Verification items for this drawing (mm, ordinates from the low corner). A direction names the side the tool comes from. Give positions to 0.01 mm unless a question says otherwise; leave off trailing zeros. Order: outer loops, then holes, each group sorted by start corner. A loop starts at its lowest first (then second) coordinate and runs counter-clockwise, first axis right, second up.
(1) Mould release check, pull along X, two halves, no side actions. Record for the marked faces 1, 2 and 3: pulls with the +X half, pulls with the -X half, needs draft (parallel to the pull), parting line crosses it, or undercut.
(2) Access from +Z, -Z, +X, -X, +Y, -Y to the whole of each face (thin tool, end or side, straight path). Record for the marked faces 4, 5 and 6.
(3) Gauge pin test, flat ends, axial feed: pin 1 (10 mm diameter, centred on x = 6.5, z = 13.5, fed in from -Y); pin 2 (1.2 mm diameter, centred on x = 13.5, y = 23.5, fed in from +Z); pin 3 (2 mm diameter, centred on x = 1, y = 33, fed in from +Z). Record the tip position at first contact, or that the pin passes through.
(4) Sectioned sample at B-B on z = 19. Record the cut outline in (x, y).
(5) Sectioned sample at A-A on y = 29. Record the cut outline in (x, z), plus the area to 3 significant figures.
(6) Sectioned sample at C-C on y = 24. Record the cut outline in (x, z).
(7) Scan lines: L1, parallel to Z at x = 2.7, y = 39; L2, parallel to Y at x = 3.05, z = 7; L3, parallel to X at y = 41, z = 13. Record each from-to range of solid material in increasing order.
(8) Sectioned sample at D-D on z = 23. Record the cut outline in (x, y).
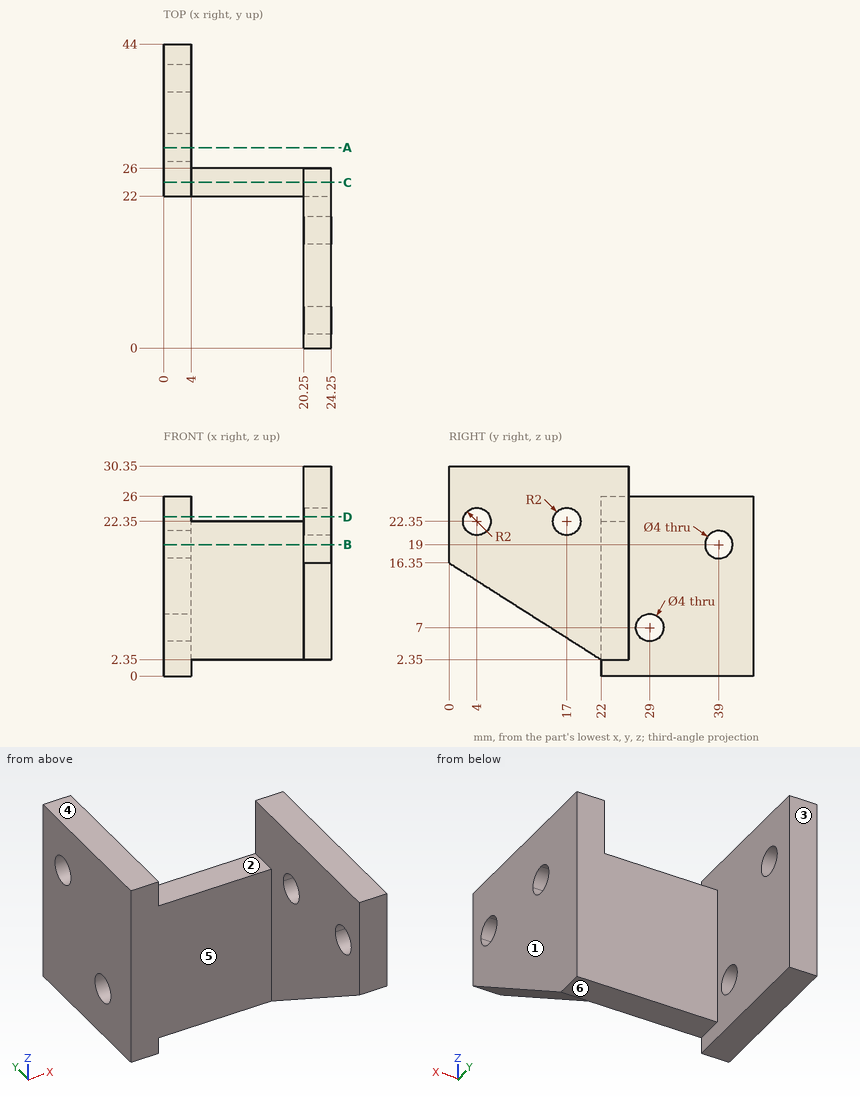
Ans:
1. face 1: pulls with the +X half
1. face 2: undercut
1. face 3: needs draft
2. face 4: +Z, -X, +Y, -Y
2. face 5: +Z, -Z, -X, -Y
2. face 6: -Z, +X, +Y, -Y
3. pin 1: stops at y = 22
3. pin 2: stops at z = 22.35
3. pin 3: stops at z = 26
4. outline: (0, 22) - (20.25, 22) - (20.25, 0) - (24.25, 0) - (24.25, 26) - (4, 26) - (4, 37) - (0, 37) - close; (0, 41) - (4, 41) - (4, 44) - (0, 44) - close
5. outline: (0, 0) - (4, 0) - (4, 5) - (0, 5) - close; (0, 9) - (4, 9) - (4, 26) - (0, 26) - close
5. area: 88.0 mm2
6. outline: (0, 0) - (4, 0) - (4, 2.35) - (24.25, 2.35) - (24.25, 30.35) - (20.25, 30.35) - (20.25, 22.35) - (4, 22.35) - (4, 26) - (0, 26) - close
7. L1: z = 0 to 17, 21 to 26
7. L2: y = 22 to 27, 31 to 44
7. L3: x = 0 to 4
8. outline: (0, 22) - (4, 22) - (4, 44) - (0, 44) - close; (20.25, 0) - (24.25, 0) - (24.25, 2.11) - (20.25, 2.11) - close; (20.25, 5.89) - (24.25, 5.89) - (24.25, 15.11) - (20.25, 15.11) - close; (20.25, 18.89) - (24.25, 18.89) - (24.25, 26) - (20.25, 26) - close
